Check sheet for the modelled part. Datum: model origin and axes. Units: mm. A direction names the side the tool comes from. Round coordinates to 2 decimals unless told otherwise and drop trailing zeros. Order: outer loops, then holes, each group sorted by start corner. A loop starts at its lowest first (then second) coordinate and runs counter-clockwise, first axis right, second up.
from build123d import *

# Parameters (mm, degrees)
F0_W     = 31
F0_H     = 47.2
F0_R     = 1.5
F1_DEPTH = 1.2
F2_W     = 28.6
F2_H     = 29
F3_DEPTH = 2.8
F4_W     = 28.2
F4_H     = 2.6
F5_DEPTH = 25
F7_DEPTH = 0.2


with BuildPart() as f1:
    # F0 (on Top) → F1 (new body)
    with BuildSketch(Plane.XY):
        Rectangle(F0_W, F0_H)
        with Locations((-12.9, 21.4)):
            Circle(F0_R, mode=Mode.SUBTRACT)
        with Locations((12.9, 21.4)):
            Circle(F0_R, mode=Mode.SUBTRACT)
    extrude(amount=F1_DEPTH)

    # F2 (on face) → F3 (join)
    with BuildSketch(Plane.XY.offset(1.2)):
        with Locations((0, -14.446534)):
            Rectangle(F2_W, F2_H)
    extrude(amount=F3_DEPTH)

    # F4 (on face) → F5 (cut)
    with BuildSketch(Plane.XZ.offset(28.946534)):
        with Locations((0, 2.5)):
            Rectangle(F4_W, F4_H)
    extrude(amount=-F5_DEPTH, mode=Mode.SUBTRACT)

    # F6 (on face) → F7 (cut, through all)
    with BuildSketch(Plane.XY.offset(4)):
        with BuildLine():
            Line((-10.05, -28.946534), (10.05, -28.946534))
            ThreePointArc((10.05, -28.946534), (0, -18.896534), (-10.05, -28.946534))
        make_face()
    extrude(amount=-F7_DEPTH, mode=Mode.SUBTRACT)


solid = f1.part
1) Draft check along Z on faces 1 (the face through (0, -14, 1.2)), 2 (the face through (0, 0.053, 3)), 3 (the face through (0, 0, 0)). Enter one of: pulls with the +Z half, pulls with the -Z half, needs draft (parallel to the pull), parting line crosses it, or undercut.
2) Sectioned sample at A-A on x = -12. Record the cut outline in (y, z), and give its area (3 significant figures).
3) Scan lines: line 1 (Z direction, x = -3.5, y = -12); line 2 (Y direction, x = 12.9, z = 0.95); line 3 (X direction, y = -4, z = 1.5). Record each from-to range of solid material in increasing order.
4) Set-up check for faces 4 (the face through (-14.3, -15, 3)), 5 (the face through (14.1, -17, 2)), 6 (the face through (14.3, -15, 3)), 7 (the face through (0, -11, 4)), 8 (the face through (0, -23.6, 1)): record each of +Z, -Z, +X, -X, +Y, -Y from which the full face is reachable in a straight line by a thin tool's end or side.
5) Gauge pin test, flat ends, axial feed: pin 1 (1.3 mm diameter, centred on x = -6, z = 0.5, fed in from -Y); pin 2 (0.8 mm diameter, centred on x = 0.5, z = 2, fed in from -Y); pin 3 (3.5 mm diameter, centred on x = -12.9, y = 21.4, fed in from +Z); pin 4 (9.5 mm diameter, centred on x = -0.5, y = 4, fed in from +Z). Record the tip position at first contact, or that the pin passes through.
6) Sectioned sample at C-C on z = 2.5. Record the cut outline in (x, y), and give its area (3 significant figures).
7) Sectioned sample at D-D on y = -2.5. Record the cut outline in (x, z), and give its area (3 significant figures).
8) Sectioned sample at B-B on y = 21.4. Record the cut outline in (x, z), and give its area (3 significant figures).
Values found:
1. face 1: undercut
1. face 2: needs draft
1. face 3: pulls with the -Z half
2. outline: (-28.95, 3.8) - (-3.95, 3.8) - (-3.95, 1.2) - (-23.6, 1.2) - (-23.6, 0) - (20.2, 0) - (20.2, 1.2) - (0.05, 1.2) - (0.05, 4) - (-28.95, 4) - close; (22.6, 0) - (23.6, 0) - (23.6, 1.2) - (22.6, 1.2) - close
2. area: 70.0 mm2
3. line 1: z = 0 to 1.2, 3.8 to 4
3. line 2: y = -23.6 to 19.9, 22.9 to 23.6
3. line 3: x = -14.3 to -14.1, 14.1 to 14.3
4. face 4: +Z, -X, +Y, -Y
4. face 5: -Y
4. face 6: +Z, +X, +Y, -Y
4. face 7: +Z, +X, -X, +Y, -Y
4. face 8: -Z, +X, -X, -Y
5. pin 1: stops at y = -23.6
5. pin 2: stops at y = -3.95
5. pin 3: stops at z = 1.2
5. pin 4: stops at z = 4
6. outline: (-14.3, -28.95) - (-14.1, -28.95) - (-14.1, -3.95) - (14.1, -3.95) - (14.1, -28.95) - (14.3, -28.95) - (14.3, 0.05) - (-14.3, 0.05) - close
6. area: 124 mm2
7. outline: (-15.5, 0) - (15.5, 0) - (15.5, 1.2) - (14.3, 1.2) - (14.3, 4) - (-14.3, 4) - (-14.3, 1.2) - (-15.5, 1.2) - close
7. area: 117 mm2
8. outline: (-15.5, 0) - (-14.4, 0) - (-14.4, 1.2) - (-15.5, 1.2) - close; (-11.4, 0) - (11.4, 0) - (11.4, 1.2) - (-11.4, 1.2) - close; (14.4, 0) - (15.5, 0) - (15.5, 1.2) - (14.4, 1.2) - close
8. area: 30.0 mm2
